from build123d import *

# Parameters (mm, degrees)
A_BASE_T_START                 = -1.5
A_BASE_T_OUTLINE_R             = 47
A_BASE_T_OUTLINE_R_2           = 1
A_BASE_T_DEPTH                 = 3
OUTER_RING_DEPTH               = 3
OUTER_RING_DEPTH_BACK          = 3
SKETCH1_R                      = 50
SKETCH1_R_2                    = 47.000000000000014
SERVO_FRAME_DEPTH              = 3
PATCHING_START                 = -3
SKETCH4_R                      = 1.000000000000005
SKETCH4_R_2                    = 0.9999999999999875
SKETCH4_R_3                    = 1.0000000000000018
PATCHING_DEPTH                 = 3
BOTTOM_HOLES_DEPTH             = 71.77428911688199
SERVO_FRAME_EXTENSION_DEPTH    = 5
F_8_0_199_DIAMETER_HOLE1_D     = 5.0546
F_8_0_199_DIAMETER_HOLE1_DEPTH = 10
F_8_0_199_DIAMETER_HOLE1_TIP   = 1.5185550424683532
SHELL_TAB_DEPTH                = 3
SHELL_TAB_EXTENSION_DEPTH      = 5
CONTOURING_R                   = 1


# Read off the part's stored shape, not the designer's step: a_base_t
with BuildPart() as part:
    # a_base_t outline → a_base_t (new body)
    with BuildSketch(Plane(origin=(0, 0, 0), x_dir=(1, 0, 0), z_dir=(0, 1, 0)).offset(A_BASE_T_START)):
        Circle(A_BASE_T_OUTLINE_R)
        with Locations((-17.009259258, -38.128042167)):
            Circle(A_BASE_T_OUTLINE_R_2, mode=Mode.SUBTRACT)
        with Locations((-9.166666665, -28.284271247)):
            Circle(A_BASE_T_OUTLINE_R_2, mode=Mode.SUBTRACT)
        with Locations((17.009259258, -38.128042167)):
            Circle(A_BASE_T_OUTLINE_R_2, mode=Mode.SUBTRACT)
        with Locations((27.5, -28.284271247)):
            Circle(A_BASE_T_OUTLINE_R_2, mode=Mode.SUBTRACT)
        with Locations((-27.5, 28.284271247)):
            Circle(A_BASE_T_OUTLINE_R_2, mode=Mode.SUBTRACT)
        with Locations((-17.009259258, 38.128042167)):
            Circle(A_BASE_T_OUTLINE_R_2, mode=Mode.SUBTRACT)
        with Locations((9.166666665, 28.284271247)):
            Circle(A_BASE_T_OUTLINE_R_2, mode=Mode.SUBTRACT)
        with Locations((17.009259258, 38.128042167)):
            Circle(A_BASE_T_OUTLINE_R_2, mode=Mode.SUBTRACT)
    extrude(amount=A_BASE_T_DEPTH)

    # Sketch1 → Outer Ring (add, two sides: drawn at the far end of the back side and taken through both)
    with BuildSketch(Plane(origin=(0, 1.5, 0), x_dir=(1, 0, 0), z_dir=(0, 1, 0)).offset(-OUTER_RING_DEPTH_BACK)):
        with Locations(Location((0, 0, 0), (0, 0, 270))):
            Circle(SKETCH1_R)
        with Locations(Location((0, 0, 0), (0, 0, 270))):
            Circle(SKETCH1_R_2, mode=Mode.SUBTRACT)
    extrude(amount=OUTER_RING_DEPTH + OUTER_RING_DEPTH_BACK)

    # Sketch2 → Servo Frame (add)
    with BuildSketch(Plane(origin=(0, 1.5, 0), x_dir=(1, 0, 0), z_dir=(0, 1, 0))):
        with BuildLine():
            Line((-38.0591968031926, -27.57711984047382), (-35.959340758040334, -26.89657621793413))
            Line((-35.959340758040334, -26.89657621793413), (-34.26367139752046, -32.128660450798996))
            Line((-34.26367139752046, -32.128660450798996), (-29.982875206994592, -30.74129461037364))
            Line((-29.982875206994592, -30.74129461037364), (-31.678544567514475, -25.509210377508683))
            Line((-31.678544567514475, -25.509210377508683), (-7.896343509037404, -17.801622375145534))
            Line((-7.896343509037404, -17.801622375145534), (-6.200674148517496, -23.033706608010526))
            Line((-6.200674148517496, -23.033706608010526), (-1.9198779579916272, -21.64634076758515))
            Line((-1.9198779579916272, -21.64634076758515), (-3.6155473185115334, -16.414256534720167))
            Line((-3.6155473185115334, -16.414256534720167), (-0.7616831914942761, -15.489345974436619))
            Line((-0.7616831914942761, -15.489345974436619), (1.8588967293091871, -23.57529433431882))
            Line((1.8588967293091871, -23.57529433431882), (-8.1296277152512, -26.812481295311326))
            Line((-8.1296277152512, -26.812481295311326), (-9.825297075771067, -21.580397062446362))
            Line((-9.825297075771067, -21.580397062446362), (-27.89976988021365, -27.438163944242362))
            Line((-27.89976988021365, -27.438163944242362), (-26.20410051969376, -32.670248177107304))
            Line((-26.20410051969376, -32.670248177107304), (-31.900225974204588, -34.516308939321476))
            ThreePointArc((-31.900225974204588, -34.516308939321476), (-35.15136263609195, -31.199065768480295), (-38.0591968031926, -27.57711984047382))
        make_face()
        with BuildLine():
            Line((-12.323065195039092, 20.183955613279007), (-22.311589639599458, 16.946768652286423))
            Line((-22.311589639599458, 16.946768652286423), (-20.615920279079525, 11.714684419421493))
            Line((-20.615920279079525, 11.714684419421493), (-38.690393083522096, 5.856917537625489))
            Line((-38.690393083522096, 5.856917537625489), (-40.38606244404183, 11.089001770490507))
            Line((-40.38606244404183, 11.089001770490507), (-46.08218789855281, 9.242941008276162))
            ThreePointArc((-46.08218789855281, 9.242941008276162), (-46.769478259318326, 4.649290628811158), (-46.999998885933856, 0.01023338735953519))
            Line((-46.999998885933856, 0.01023338735953519), (-44.90014284078164, 0.6907770098992967))
            Line((-44.90014284078164, 0.6907770098992967), (-46.595812201301534, 5.922861242764241))
            Line((-46.595812201301534, 5.922861242764241), (-42.31501601077568, 7.31022708318961))
            Line((-42.31501601077568, 7.31022708318961), (-40.61934665025577, 2.0781428503246593))
            Line((-40.61934665025577, 2.0781428503246593), (-16.8371455917787, 9.785730852687836))
            Line((-16.8371455917787, 9.785730852687836), (-18.53281495229861, 15.017815085552826))
            Line((-18.53281495229861, 15.017815085552826), (-14.252018761772744, 16.405180925978193))
            Line((-14.252018761772744, 16.405180925978193), (-12.556349401252827, 11.173096693113212))
            Line((-12.556349401252827, 11.173096693113212), (-9.702485274235583, 12.09800725339679))
            Line((-9.702485274235583, 12.09800725339679), (-12.323065195039092, 20.183955613279007))
        make_face()
    extrude(amount=SERVO_FRAME_DEPTH)

    # Sketch4 → Patching (add)
    with BuildSketch(Plane(origin=(0, 1.5, 0), x_dir=(1, 0, 0), z_dir=(0, 1, 0)).offset(PATCHING_START)):
        with Locations((-9.166666664999994, -28.284271247461895)):
            Circle(SKETCH4_R)
        with Locations((27.499999999999897, -28.284271247461895)):
            Circle(SKETCH4_R_2)
        with Locations((-27.499999999999897, 28.284271247461895)):
            Circle(SKETCH4_R_3)
        with Locations((9.166666664999994, 28.284271247461895)):
            Circle(SKETCH4_R)
    extrude(amount=PATCHING_DEPTH)

    # Sketch3 → Bottom Holes (cut, through all)
    with BuildSketch(Plane(origin=(0, 1.5, 0), x_dir=(1, 0, 0), z_dir=(0, 1, 0))):
        Polygon((-2.4573525520141377, -10.257261741571627), (-8.006815913715702, 6.865923020531821), (3.8842846155226813, 10.719717021713405), (9.43374797722423, -6.403467740390065), align=None)
        Polygon((11.007812758181103, 21.175234550786502), (8.078929317282705, 30.212470953007827), (3.084667095002796, 28.593877472511632), (2.6992876948846334, 29.78298752543549), (-6.337948707336641, 26.854104084537454), (-5.952569307218477, 25.6649940316136), (-10.9468315294987, 24.046400551117266), (-8.017948088600651, 15.009164148896), (-3.023685866320578, 16.62775762939225), (-2.6383064662022653, 15.438647576468425), (6.398929936019005, 18.36753101736646), (6.01355053590084, 19.55664107029031), align=None)
        Polygon((19.270601899965627, -21.348744750290177), (19.65598130008379, -22.53785480321403), (10.618744897862516, -25.46673824411206), (10.233365497744353, -24.27762819118821), (5.239103275464198, -25.89622167168446), (2.3102198345661495, -16.85898526946319), (7.304482056846301, -15.240391788966894), (6.9191026567281435, -14.051281736043038), (15.95633905894941, -11.122398295145004), (16.34171845906757, -12.31150834806886), (21.335980681347763, -10.692914867572457), (24.2648641222456, -19.7301512697939), align=None)
    extrude(amount=-BOTTOM_HOLES_DEPTH, mode=Mode.SUBTRACT)

    # Sketch8 → Servo Frame Extension (add)
    with BuildSketch(Plane(origin=(0, 4.500000000000001, 0), x_dir=(1, 0, 0), z_dir=(0, 1, 0))):
        Polygon((1.8588967293091865, -23.57529433431882), (-0.7616831914942761, -15.489345974436619), (-3.6155473185115334, -16.414256534720167), (-1.9198779579916272, -21.64634076758515), (-6.200674148517496, -23.033706608010526), (-7.896343509037404, -17.801622375145534), (-31.678544567514475, -25.509210377508683), (-29.982875206994592, -30.74129461037364), (-29.057964646711014, -33.59515873739088), (-26.20410051969376, -32.670248177107304), (-27.89976988021365, -27.438163944242362), (-9.825297075771067, -21.580397062446362), (-8.1296277152512, -26.812481295311326), align=None)
        Polygon((-40.38606244404183, 11.089001770490507), (-43.23992657105916, 10.164091210206845), (-42.31501601077568, 7.31022708318961), (-40.61934665025577, 2.0781428503246593), (-16.837145591778697, 9.785730852687836), (-18.53281495229861, 15.017815085552826), (-14.252018761772744, 16.405180925978193), (-12.556349401252827, 11.173096693113212), (-9.702485274235583, 12.09800725339679), (-12.323065195039092, 20.183955613279007), (-22.311589639599458, 16.946768652286423), (-20.615920279079525, 11.714684419421493), (-38.690393083522096, 5.856917537625489), align=None)
    extrude(amount=SERVO_FRAME_EXTENSION_DEPTH)

    # #8 (0.199) Diameter Hole1
    with Locations(Plane(origin=(0, 1.5, 0), x_dir=(1, 0, 0), z_dir=(0, 1, 0))):
        with Locations((17.009259258, -38.128042167), (17.009259258, 38.128042167), (-17.009259258, 38.128042167), (-17.009259258, -38.128042167)):
            Hole(F_8_0_199_DIAMETER_HOLE1_D / 2, depth=F_8_0_199_DIAMETER_HOLE1_DEPTH)
            with Locations((0, 0, -(F_8_0_199_DIAMETER_HOLE1_DEPTH + F_8_0_199_DIAMETER_HOLE1_TIP / 2))):  # 118° drill point
                Cone(0, F_8_0_199_DIAMETER_HOLE1_D / 2, F_8_0_199_DIAMETER_HOLE1_TIP, mode=Mode.SUBTRACT)

    # Sketch21 → Shell Tab (add)
    with BuildSketch(Plane(origin=(0, 1.5, 0), x_dir=(1, 0, 0), z_dir=(0, 1, 0))):
        with BuildLine():
            Line((38.43738005388435, 4.573146492125436), (46.4498888135124, 7.169925328225916))
            ThreePointArc((46.4498888135124, 7.169925328225916), (44.71053798993682, 14.490265444442931), (41.825336012094446, 21.439245963312132))
            Line((41.825336012094446, 21.439245963312132), (33.81282725246639, 18.842467127211638))
            ThreePointArc((33.81282725246639, 18.842467127211638), (39.954097778241405, 12.948747843970278), (38.43738005388435, 4.573146492125436))
        make_face()
    extrude(amount=SHELL_TAB_DEPTH)

    # Sketch22 → Shell Tab Extension (add)
    with BuildSketch(Plane(origin=(0, 4.500000000000001, 0), x_dir=(1, 0, 0), z_dir=(0, 1, 0))):
        with BuildLine():
            Line((38.43738005388435, 4.573146492125436), (42.61596967836049, 5.927388144410685))
            ThreePointArc((42.61596967836049, 5.927388144410685), (42.80796190525865, 13.873658404253868), (37.99141687694254, 20.19670877949689))
            Line((37.99141687694254, 20.19670877949689), (33.81282725246639, 18.842467127211638))
            ThreePointArc((33.81282725246639, 18.842467127211638), (39.954097778241405, 12.948747843970278), (38.43738005388435, 4.573146492125436))
        make_face()
    extrude(amount=SHELL_TAB_EXTENSION_DEPTH)

    # Contouring
    contouring_edges = [part.edges().sort_by_distance(p)[0] for p in [
        (33.81282725246639, 5.5, -18.84246712721164),
        (38.43738005388435, 5.5, -4.573146492125435),
        (46.44988881351241, 3, -7.169925328225917),
        (41.82533601209445, 3, -21.439245963312132),
        (42.61596967836049, 7.000000000000001, -5.927388144410685),
        (37.99141687694254, 7.000000000000001, -20.19670877949689),
    ]]
    fillet(contouring_edges, radius=CONTOURING_R)


solid = part.part
CAD build for the part. Positions are in the model's coordinates, mm. A direction names the side the tool comes from. Coordinates: 2 decimals unless noted, no trailing zeros. Loops run counter-clockwise (first coordinate to the right, second up) from the corner with the lowest first, then second, coordinate; pieces in that order, holes last. Notation, with made-up numbers: (77, -32.75) -> (88, -32.75) arc R13 cw to (88, -21.75) -> close; hole circle Ø4 at (-0.5, 7). An arc over 180 degrees is marked (long way). One line per item, written item: value.
1. Slice it at A-A on y = 0. Give the number of separate pieces and of enclosed holes in the cut face, and give its area (3 significant figures).
Answers:
separate pieces: 1
enclosed holes: 7
area: 7,120 mm^2
2. Slice it at D-D on z = 42. Write the cut outline in (x, y), and give its area (3 significant figures).
Answers:
outline: (-27.13, -1.5) -> (27.13, -1.5) -> (27.13, 4.5) -> (21.1, 4.5) -> (21.1, 1.5) -> (-21.1, 1.5) -> (-21.1, 4.5) -> (-27.13, 4.5) -> close
area: 199 mm^2
3. Drill centre lines: line 1 (Y direction, x = 0.5, z = 13); line 2 (Z direction, x = -8, y = 3.75); line 3 (Z direction, x = 17.5, y = 2). Where is each one in solid material? Low to high. Write a range as [from, to].
Answers:
line 1: y = [-1.5, 1.5]
line 2: z = [-49.36, -46.31], [17.84, 26.77], [46.31, 49.36]
line 3: z = [-46.84, -43.62], [43.62, 46.84]
4. Pull direction Z, two halves, no side cores. Call faces 4 (the face through (15.02, 1.46, 47.69)), 5 (the face through (-29.4, 4.5, 33.1)), 6 (the face through (-4.03, 5.44, 22.33)): pulls with the +Z half, pulls with the -Z half, needs draft (parallel to the pull), parting line crosses it, or undercut.
Answers:
face 4: parting line crosses it
face 5: needs draft
face 6: undercut
5. Flat gauge pins, fed straight in: P1, Ø4, axis at y = 6, z = 36, coming from the +X side; P2, Ø5, axis at y = 0.5, z = -31, coming from the +X side; P3, Ø8, axis at x = 17.01, z = -38.13, coming from the +Y side. Where does each tip first touch, or does it go through?
Answers:
P1: stops at x = 36.02
P2: stops at x = 41.08
P3: stops at y = 1.5
6. Slice it at B-B on x = 33.5. Write the cut outline in (y, z), and give its area (3 significant figures).
Answers:
outline: (-1.5, -37.12) -> (4.5, -37.12) -> (4.5, -32.97) -> (1.5, -32.97) -> (1.5, 32.97) -> (4.5, 32.97) -> (4.5, 37.12) -> (-1.5, 37.12) -> close
area: 248 mm^2
7. Which spindle directions (+Z, -Z, +X, -X, +Y, -Y) get a long thin tool onto all of the face, cutting with end or side? Do faces 1 (the face through (-44.5, 3, -6.6)), 2 (the face through (42.84, 6.96, -13.77)), 3 (the face through (4.77, 0.02, 16.06)). Say none if no direction does.
Answers:
face 1: +Y
face 2: +X, +Y
face 3: +Y, -Y
